The drawing under review shows one solid part. Ordinate dimensions are in mm from its lowest x, y, z. A direction names the side the tool comes from. Give positions to 0.01 mm unless a question says otherwise; leave off trailing zeros. Write each loop counter-clockwise with the first axis right and the second up, starting at its lowest first coordinate (ties: lowest second). Pieces come first, ordered by that corner, then holes. Notation, with made-up numbers: (27.5, -19) -> (39.5, -19) arc R16 ccw to (39.5, -15) -> close; hole circle Ø5 at (24.5, 51.25). An arc over 180 degrees is marked (long way). Put each result on its own line as item: value. Start each with the question number.
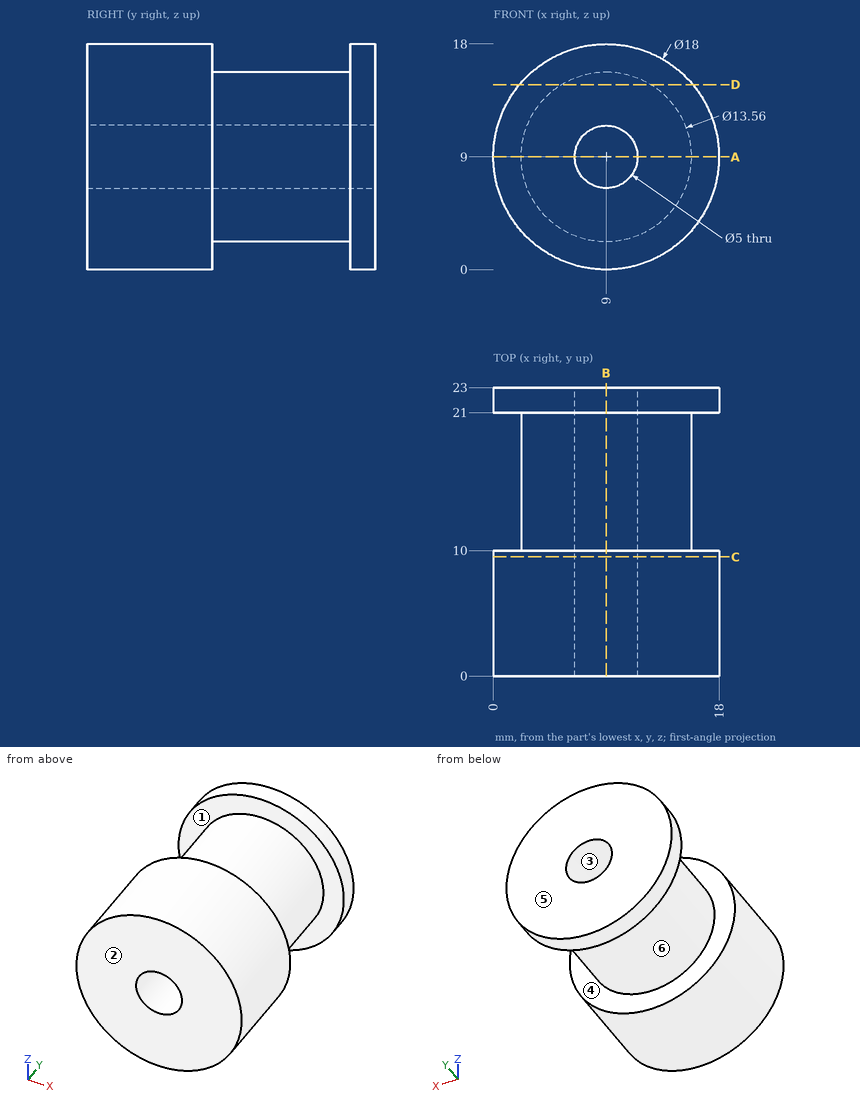
Q1. Take a section at D-D on z = 14.75. Give the boundary of the cut face in (x, y).
Q2. For pin 1 (2 mm diameter, centred on x = 10, z = 9.5, fed in from -Y); pin 2 (10 mm diameter, centred on y = 10, z = 15.5, fed in from +X); pin 3 (6 mm diameter, centred on y = 15.5, z = 7.5, fed in from +X); pin 4 (1.5 mm diameter, centred on y = 13.5, z = 14, fed in from -X), all flat-tipped, find the tip position at first contact; note any pin that passes through.
Q3. Take a section at C-C on y = 9.5. Give the boundary of the cut face in (x, z), then the cut area to 3 significant figures.
Q4. Take a section at B-B on x = 9. Give the boundary of the cut face in (y, z), then the cut area to 3 significant figures.
Q5. Machinability: for the marked faces 1 and 2, which of the approach directions +Z, -Z, +X, -X, +Y, -Y give a long, thin tool a straight path to every point of the face, cutting with its end or side? Answer none if there is none.
Q6. Mouldability with a two-part tool opening along Y and no side actions: class the marked faces 3, 4, 5 and 6 as +Y half, -Y half, draft (parallel to the pull), parting line (faces both ways), or undercut.
Q7. To check wall thickness, follow probe 1 along X at (y, z) = (5.25, 9); probe 2 along Y at (x, z) = (15.75, 14); probe 3 along X at (y, z) = (12.75, 9). State the ranges of each line that lie inside material, in increasing order. Write a range as from..to.
Q8. Take a section at A-A on z = 9. Give the boundary of the cut face in (x, y).
Result:
1. outline: (2.08, 0) -> (15.92, 0) -> (15.92, 10) -> (12.59, 10) -> (12.59, 21) -> (15.92, 21) -> (15.92, 23) -> (2.08, 23) -> (2.08, 21) -> (5.41, 21) -> (5.41, 10) -> (2.08, 10) -> close
2. pin 1: passes through
2. pin 2: stops at x = 17.87
2. pin 3: stops at x = 15.78
2. pin 4: stops at x = 3.72
3. outline: circle Ø18 at (9, 9); hole circle Ø5 at (9, 9)
3. area: 235 mm^2
4. outline: (0, 0) -> (10, 0) -> (10, 2.22) -> (21, 2.22) -> (21, 0) -> (23, 0) -> (23, 6.5) -> (0, 6.5) -> close; (0, 11.5) -> (23, 11.5) -> (23, 18) -> (21, 18) -> (21, 15.78) -> (10, 15.78) -> (10, 18) -> (0, 18) -> close
4. area: 250 mm^2
5. face 1: none
5. face 2: +Z, -Z, +X, -X, -Y
6. face 3: draft
6. face 4: undercut
6. face 5: +Y half
6. face 6: undercut
7. probe 1: x = 0..6.5, 11.5..18
7. probe 2: y = 0..10, 21..23
7. probe 3: x = 2.22..6.5, 11.5..15.78
8. outline: (0, 0) -> (6.5, 0) -> (6.5, 23) -> (0, 23) -> (0, 21) -> (2.22, 21) -> (2.22, 10) -> (0, 10) -> close; (11.5, 0) -> (18, 0) -> (18, 10) -> (15.78, 10) -> (15.78, 21) -> (18, 21) -> (18, 23) -> (11.5, 23) -> close
